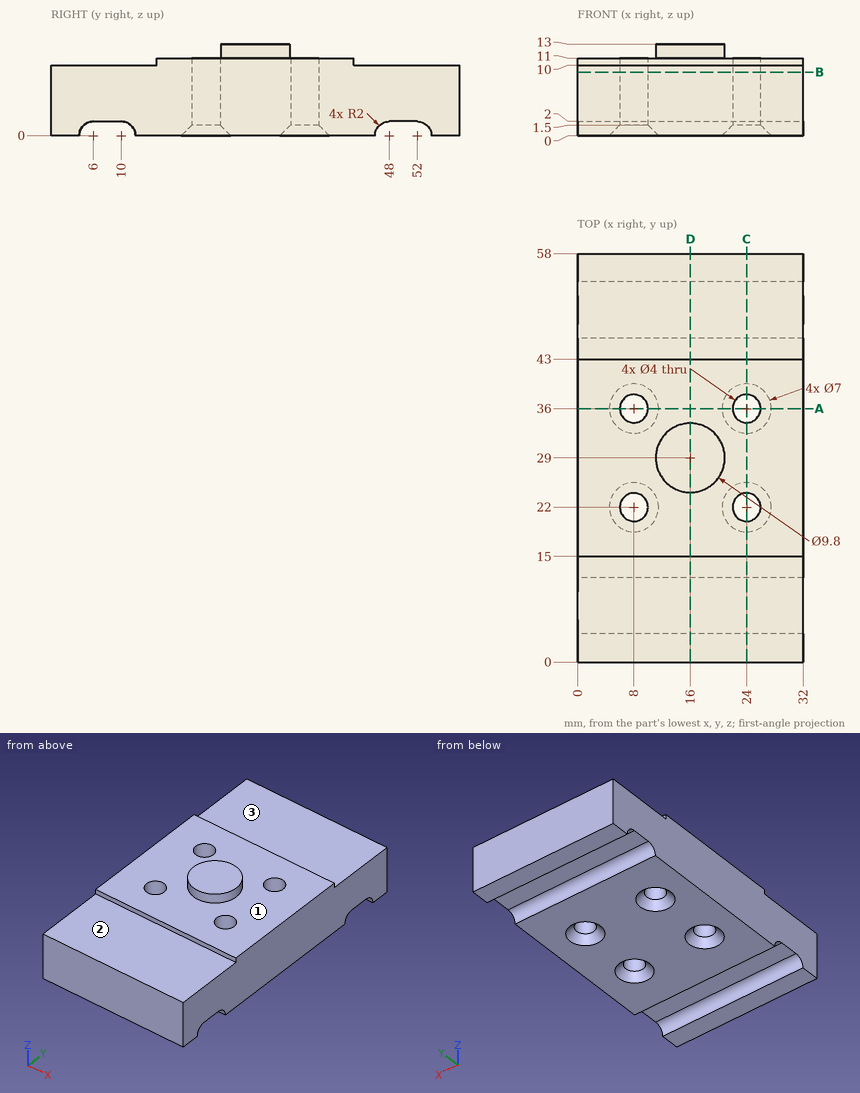
Source: three-view drawing plus pictorial views. Frame: mm from the lowest corner of the part. A direction names the side the tool comes from. Give positions to 0.01 mm unless a question says otherwise; leave off trailing zeros. Order: outer loops, then holes, each group sorted by start corner. A loop starts at its lowest first (then second) coordinate and runs counter-clockwise, first axis right, second up. Notation, with made-up numbers: (65, -27) -> (73, -27) arc R21 cw to (73, 1) -> close; hole circle Ø11 at (18.25, -9). An arc over 180 degrees is marked (long way). Put each result on its own line as item: value.
Q1. Reachability of the marked faces 1, 2 and 3 from +Z, -Z, +X, -X, +Y, -Y: full face, straight path, thin tool, end or side. Return the list, or none.
Here are the results:
face 1: +Z
face 2: +Z, +X, -X, -Y
face 3: +Z, +X, -X, +Y
Q2. Section C-C, the plane x = 24. Return loops of the section in (y, z), then the cut area to 3 significant figures.
Here are the results:
outline: (0, 0) -> (4, 0) arc R2 cw to (6, 2) -> (10, 2) arc R2 cw to (12, 0) -> (18.5, 0) -> (20, 1.5) -> (20, 11) -> (15, 11) -> (15, 10) -> (0, 10) -> close; (24, 1.5) -> (25.5, 0) -> (32.5, 0) -> (34, 1.5) -> (34, 11) -> (24, 11) -> close; (38, 1.5) -> (39.5, 0) -> (46, 0) arc R2 cw to (48, 2) -> (52, 2) arc R2 cw to (54, 0) -> (58, 0) -> (58, 10) -> (43, 10) -> (43, 11) -> (38, 11) -> close
area: 487 mm^2
Q3. Section B-B, the plane z = 9. Return loops of the section in (x, y).
Here are the results:
outline: (0, 0) -> (32, 0) -> (32, 58) -> (0, 58) -> close; hole circle Ø4 at (8, 22); hole circle Ø4 at (8, 36); hole circle Ø4 at (24, 22); hole circle Ø4 at (24, 36)
Q4. Section D-D, the plane x = 16. Return loops of the section in (y, z).
Here are the results:
outline: (0, 0) -> (4, 0) arc R2 cw to (6, 2) -> (10, 2) arc R2 cw to (12, 0) -> (46, 0) arc R2 cw to (48, 2) -> (52, 2) arc R2 cw to (54, 0) -> (58, 0) -> (58, 10) -> (43, 10) -> (43, 11) -> (33.9, 11) -> (33.9, 13) -> (24.1, 13) -> (24.1, 11) -> (15, 11) -> (15, 10) -> (0, 10) -> close
Q5. Material intervals for L1, parallel to Y at x = 8, z = 5.25; L2, parallel to Y at x = 3, z = 1.5; L3, parallel to Z at x = 24, y = 14, sorted ascending.
Here are the results:
L1: y = 0 to 20, 24 to 34, 38 to 58
L2: y = 0 to 4.68, 11.32 to 46.68, 53.32 to 58
L3: z = 0 to 10
Q6. Pin query (flat end, axial travel): pin 1 (3 mm diameter, centred on x = 18, y = 50, fed in from -Z); pin 2 (6.5 mm diameter, centred on x = 24, y = 22, fed in from -Z); pin 3 (7.5 mm diameter, centred on x = 17, y = 50.5, fed in from +Z). Return the tip coordinate at first contact, or that it passes through.
Here are the results:
pin 1: stops at z = 2
pin 2: stops at z = 0.25
pin 3: stops at z = 10
Q7. Section A-A, the plane y = 36. Return loops of the section in (x, z), then the cut area to 4 significant figures.
Here are the results:
outline: (0, 0) -> (4.5, 0) -> (6, 1.5) -> (6, 11) -> (0, 11) -> close; (10, 1.5) -> (11.5, 0) -> (20.5, 0) -> (22, 1.5) -> (22, 11) -> (10, 11) -> close; (26, 1.5) -> (27.5, 0) -> (32, 0) -> (32, 11) -> (26, 11) -> close
area: 259.5 mm^2
